Read the model definition and answer for the solid it produces. Units are mm, in the model's axes. Face numbers are marked on the shaded views. A direction names the side the tool comes from. Give positions to 0.01 mm unless a question says otherwise; leave off trailing zeros. Write each loop counter-clockwise with the first axis right and the second up, starting at its lowest first coordinate (ties: lowest second). Pieces come first, ordered by that corner, then holes.
```python
from build123d import *

# Parameters (mm, degrees)
F0_W     = 49.9249994755
F0_H     = 71.728259325
F1_DEPTH = 127
F2_W     = 71.728259325
F2_H     = 93.4169888496
F3_DEPTH = 50.6314188242
F4_DEPTH = 25.4


with BuildPart() as f1:
    # F0 (on Top) → F1 (new body)
    with BuildSketch(Plane.XY):
        with Locations((-24.9624997377, -35.8641296625)):
            Rectangle(F0_W, F0_H)
    extrude(amount=F1_DEPTH)

    # F2 (on face) → F3 (join)
    with BuildSketch(Plane.YZ):
        with Locations((-35.8641296625, 46.7084944248)):
            Rectangle(F2_W, F2_H)
    extrude(amount=F3_DEPTH)

    # F4 (add): a face of the model
    f4_faces = [f1.faces().sort_by_distance(p)[0] for p in [
        (-3.4809309458, -71.728259325, 56.3257611352),
    ]]
    extrude(f4_faces, amount=F4_DEPTH)


solid = f1.part
```
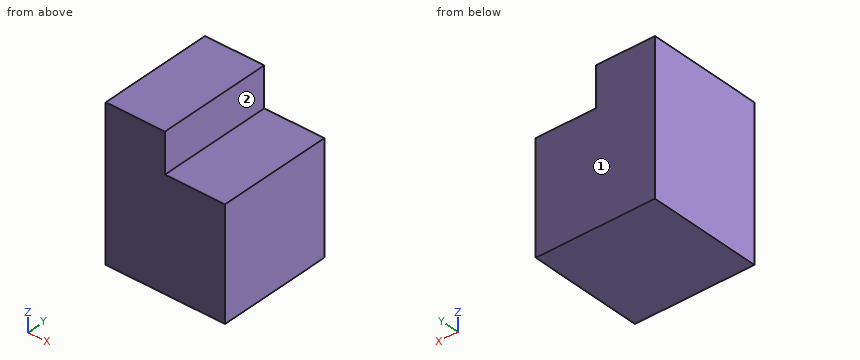
Item 1: Section B-B (x = 14) is taken. Write down the section's boundary in (y, z), and give its area (3 significant figures).
Result set:
outline: (-97.13, 0) - (0, 0) - (0, 93.42) - (-97.13, 93.42) - close
area: 9,070 mm2
Item 2: Which of the six approach directions +Z, -Z, +X, -X, +Y, -Y give full straight-line access (tool end or side, diameter ignored) to the marked faces 1 and 2?
Result set:
face 1: +Z, -Z, +X, -X, +Y
face 2: +Z, +X, +Y, -Y
Item 3: Section A-A (y = -42.5) is taken. Write down the section's boundary in (x, z) (3 decimals).
Result set:
outline: (-49.925, 0) - (50.631, 0) - (50.631, 93.417) - (0, 93.417) - (0, 127) - (-49.925, 127) - close
Item 4: Find the intervals of material crossed by line 1 along Z through (x, y) = (46, -51.5); line 2 along X through (y, z) = (-47, 117.5) (3 decimals), in increasing order.
Result set:
line 1: z = 0 to 93.42
line 2: x = -49.925 to 0
Item 5: This flat-tipped pin is pushed along its axis until it touches: pin 1 Ø8 at (x, y) = (28, -87) entering from +Z. Where does it stop, or does it pass through?
Result set:
pin 1: stops at z = 93.42
